Input: dimensioned drawing with shaded views. Units: mm. Origin: part minimum x, y, z. A direction names the side the tool comes from. Coordinates: 2 decimals unless noted, no trailing zeros. Order: outer loops, then holes, each group sorted by start corner. A loop starts at its lowest first (then second) coordinate and runs counter-clockwise, first axis right, second up. Notation, with made-up numbers: (-5, -35) - (30, -35) arc R30 cw to (30, -7) - close; hole circle Ø7 at (28, -21.75). An arc over 180 degrees is marked (long way). Answer as CSV lines item,"result". Start each with the question number.
Item 1: Section A-A (y = 70). Output: boundary loops of the cut face in (x, z), and give its area (3 significant figures).
Item 2: Access query for the marked faces 1 and 2. Directions: +Z, -Z, +X, -X, +Y, -Y. A direction counts if a zero-diameter tool reaches every point of the face in a straight line with its end or side. Return the directions, or none.
Item 3: First-contact query: pin 1 (8 mm diameter, centred on x = 55.5, z = 6.5, fed in from +Y); pin 2 (15 mm diameter, centred on y = 50, z = 22, fed in from +X). Flat tips, straight axial feed; report the tip coordinate or a pass-through.
Item 4: Section C-C (x = 7). Output: boundary loops of the cut face in (y, z).
Item 5: Section B-B (z = 25). Output: boundary loops of the cut face in (x, y), and give its area (3 significant figures).
Item 6: Material intervals for line 1 along Z through (x, y) = (6, 70); line 2 along X through (y, z) = (72.5, 43), sorted ascending.
Item 7: Section D-D (z = 33.5). Output: boundary loops of the cut face in (x, y), and give its area (3 significant figures).
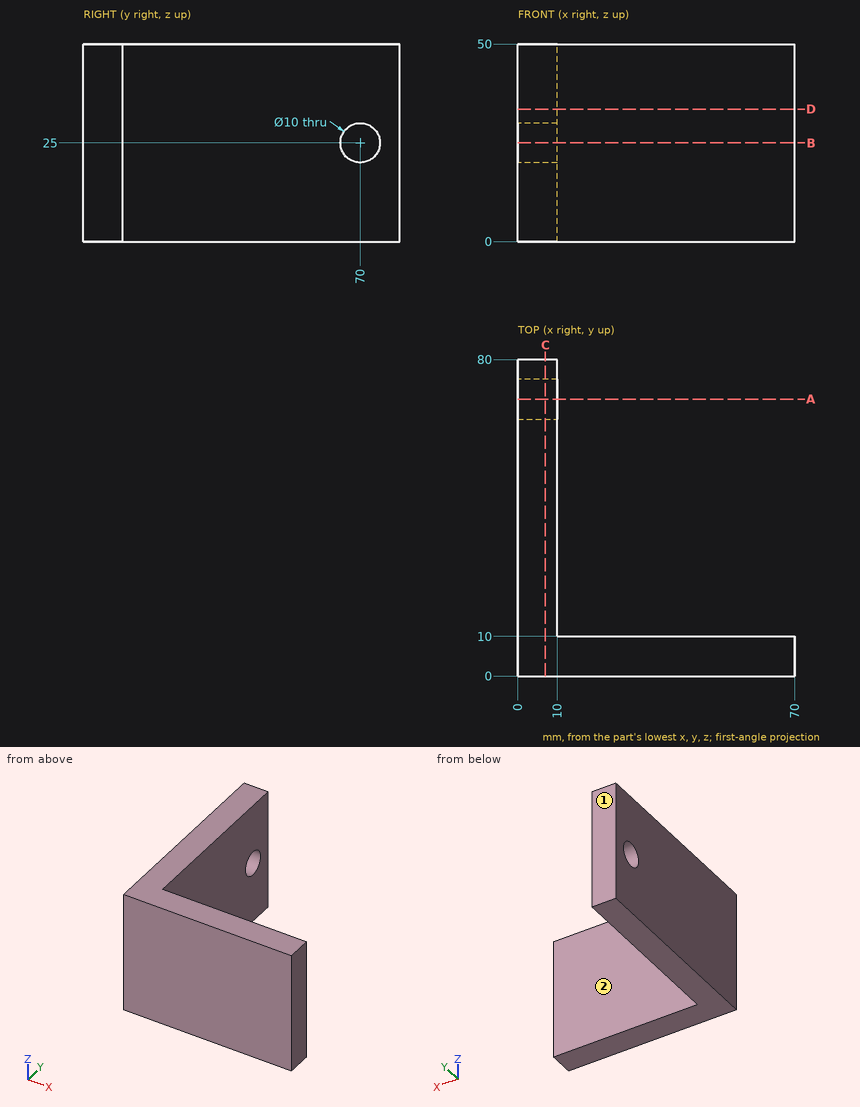
Determined:
1,outline,"(0, 0) - (10, 0) - (10, 20) - (0, 20) - close; (0, 30) - (10, 30) - (10, 50) - (0, 50) - close"
1,area,"400 mm^2"
2,face 1,"+Z, -Z, +X, -X, +Y"
2,face 2,"+Z, -Z, +X, +Y"
3,pin 1,"stops at y = 10"
3,pin 2,"stops at x = 10"
4,outline,"(0, 0) - (80, 0) - (80, 50) - (0, 50) - close; hole circle Ø10 at (70, 25)"
5,outline,"(0, 0) - (70, 0) - (70, 10) - (10, 10) - (10, 65) - (0, 65) - close; (0, 75) - (10, 75) - (10, 80) - (0, 80) - close"
5,area,"1,300 mm^2"
6,line 1,"z = 0 to 20, 30 to 50"
6,line 2,"x = 0 to 10"
7,outline,"(0, 0) - (70, 0) - (70, 10) - (10, 10) - (10, 80) - (0, 80) - close"
7,area,"1,400 mm^2"
